Geometry check sheet. Reference: the model listing, model coordinates, mm. Face numbers are marked on the shaded views. A direction names the side the tool comes from. Give positions to 0.01 mm unless a question says otherwise; leave off trailing zeros. Loops run counter-clockwise (first coordinate to the right, second up) from the corner with the lowest first, then second, coordinate; pieces in that order, holes last.
1. Cross-section at C-C, the plane x = -2. State how many separate pieces and enclosed holes the cut face has, plus the area to 3 significant figures.
2. Cross-section at A-A, the plane z = -4.6. Record the cut outline in (x, y), plus the area to 3 significant figures.
3. Cross-section at B-B, the plane y = -11.5. Record the cut outline in (x, z), plus the area to 3 significant figures.
4. Material ranges on L1, parallel to X at y = 43.25, z = -4.6; L2, parallel to Z at x = -0.75, y = -30.5; L3, parallel to Y at x = 7, z = -2.5, recorded low to high.
5. Tool access check on the marked faces 1 and 2. Record the directions out of +Z, -Z, +X, -X, +Y, -Y that give a thin tool (end or side, any length) a straight path to the whole face; none if there is none.
6. Go/stop test with flat-tipped pins: pin 1 Ø2 at (x, z) = (7.05, -4.6) entering from -Y; pin 2 Ø1.5 at (x, y) = (4, 33) entering from -Z; pin 3 Ø2.5 at (x, z) = (-0.5, -4.5) entering from -Y; pin 4 Ø6 at (x, y) = (-6, 0.5) entering from +Z. Record where each tip stops, or that it passes through.
from build123d import *

# Parameters (mm, degrees)
SKETCH1_W                    = 18.9
SKETCH1_H                    = 85
BASE_FLANGE1_DEPTH           = 1
EDGE_FLANGE1_STRIP_W         = 5.2
EDGE_FLANGE1_STRIP_H         = 1
EDGE_FLANGE1_STRIP_CUT_DEPTH = 18.9
EDGE_FLANGE1_DEPTH           = 18.9
SKETCH9_R                    = 1.4
CUT_EXTRUDE1_DEPTH           = 10
CUT_EXTRUDE4_DEPTH           = 10


# Sheet-metal steps are written as plain solids
with BuildPart() as part:
    # Sketch1 → Base-Flange1 (new body)
    with BuildSketch(Plane.XY):
        Rectangle(SKETCH1_W, SKETCH1_H)
        with BuildLine():
            Line((-5.65, -36.5), (-5.65, -38.5))
            ThreePointArc((-5.65, -38.5), (-7.05, -39.9), (-8.45, -38.5))
            Line((-8.45, -38.5), (-8.45, -36.5))
            ThreePointArc((-8.45, -36.5), (-7.05, -35.1), (-5.65, -36.5))
        make_face(mode=Mode.SUBTRACT)
        with BuildLine():
            Line((8.45, -36.5), (8.45, -38.5))
            ThreePointArc((8.45, -38.5), (7.05, -39.9), (5.65, -38.5))
            Line((5.65, -38.5), (5.65, -36.5))
            ThreePointArc((5.65, -36.5), (7.05, -35.1), (8.45, -36.5))
        make_face(mode=Mode.SUBTRACT)
    extrude(amount=-BASE_FLANGE1_DEPTH)

    # Edge-Flange1 strip (across the edge) → Edge-Flange1 strip cut (cut)
    with BuildSketch(Plane(origin=(-9.45, 42.5, -1), x_dir=(0, -1, 0), z_dir=(1, 0, 0))):
        with Locations((-2, -0.5)):
            Rectangle(EDGE_FLANGE1_STRIP_W, EDGE_FLANGE1_STRIP_H)
    extrude(amount=EDGE_FLANGE1_STRIP_CUT_DEPTH, mode=Mode.SUBTRACT)

    # Edge-Flange1 section (across the edge) → Edge-Flange1 (add)
    with BuildSketch(Plane(origin=(-9.45, 42.5, -1), x_dir=(0, -1, 0), z_dir=(1, 0, 0))):
        with BuildLine():
            Line((-1, 0.6), (-1, 6))
            Line((-1, 6), (0, 6))
            Line((0, 6), (0, 0.6))
            ThreePointArc((0, 0.6), (0.175735931, 0.175735931), (0.6, 0))
            Line((0.6, 0), (0.6, -1))
            ThreePointArc((0.6, -1), (-0.53137085, -0.53137085), (-1, 0.6))
        make_face()
    extrude(amount=EDGE_FLANGE1_DEPTH)

    # Sketch9 → Cut-Extrude1 (cut)
    with BuildSketch(Plane(origin=(0, 43.5, 0), x_dir=(1, 0, 0), z_dir=(0, 1, 0))):
        with Locations(Location((-7.05, 4.6, 0), (0, 0, 270))):
            Circle(SKETCH9_R)
        with Locations(Location((7.05, 4.6, 0), (0, 0, 270))):
            Circle(SKETCH9_R)
    extrude(amount=-CUT_EXTRUDE1_DEPTH, mode=Mode.SUBTRACT)

    # Sketch12 → Cut-Extrude4 (cut)
    with BuildSketch(Plane.XY):
        Polygon((7.45, 39.9), (-7.45, 21.9), (-7.45, 39.9), align=None)
        Polygon((7.45, 36.763509145), (-7.45, 18.763509145), (7.45, 18.763509145), align=None)
        Polygon((-7.45, 16.763509145), (7.45, 16.763509145), (-7.45, -1.236490855), align=None)
        Polygon((7.45, 13.62701829), (-7.45, -4.37298171), (7.45, -4.37298171), align=None)
        Polygon((-7.45, -6.37298171), (7.45, -6.37298171), (-7.45, -24.37298171), align=None)
        Polygon((-7.45, -27.509472565), (7.45, -9.509472565), (7.45, -27.509472565), align=None)
    extrude(amount=-CUT_EXTRUDE4_DEPTH, mode=Mode.SUBTRACT)


solid = part.part
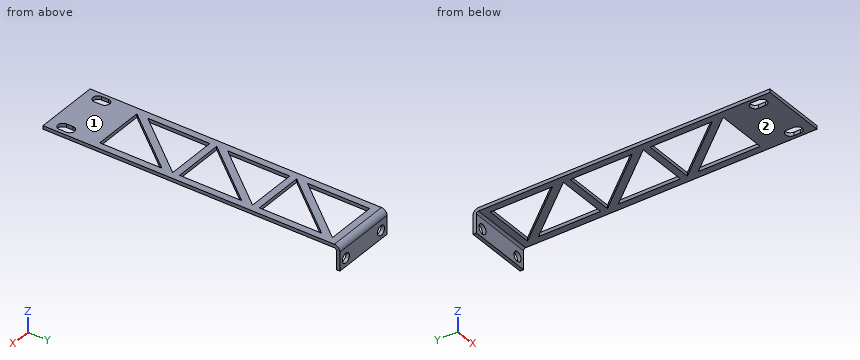
Result:
1. separate pieces: 7
1. enclosed holes: 0
1. area: 37.5 mm2
2. outline: (-9.45, 42.5) - (-8.45, 42.5) - (-8.45, 43.5) - (-9.45, 43.5) - close; (-5.65, 42.5) - (5.65, 42.5) - (5.65, 43.5) - (-5.65, 43.5) - close; (8.45, 42.5) - (9.45, 42.5) - (9.45, 43.5) - (8.45, 43.5) - close
2. area: 13.3 mm2
3. outline: (-9.45, -1) - (-7.45, -1) - (-7.45, 0) - (-9.45, 0) - close; (3.21, -1) - (5.8, -1) - (5.8, 0) - (3.21, 0) - close; (7.45, -1) - (9.45, -1) - (9.45, 0) - (7.45, 0) - close
3. area: 6.60 mm2
4. L1: x = -9.45 to -8.45, -5.65 to 5.65, 8.45 to 9.45
4. L2: z = -1 to 0
4. L3: y = 42.5 to 43.5
5. face 1: +Z, +X, -X, +Y, -Y
5. face 2: -Z, +X, -X, -Y
6. pin 1: passes through
6. pin 2: stops at z = -1
6. pin 3: stops at y = 42.5
6. pin 4: stops at z = 0
